Verification items for the finished model (mm, model axes). A direction names the side the tool comes from. Round coordinates to 2 decimals unless told otherwise and drop trailing zeros. Order: outer loops, then holes, each group sorted by start corner. A loop starts at its lowest first (then second) coordinate and runs counter-clockwise, first axis right, second up.
```python
from build123d import *

# Parameters (mm, degrees)
F0_R      = 3.5
F1_DEPTH  = 1.5
F2_R      = 2.5
F3_DEPTH  = 1
F4_R      = 3.5
F4_R_2    = 2.5
F5_DEPTH  = 1.5
F6_R      = 1
F7_R      = 1
F10_R     = 3.5
F11_DEPTH = 1.5
F12_R     = 1
F13_D     = 3.5


with BuildPart() as f1:
    # F0 (on Front) → F1 (new body)
    with BuildSketch(Plane.XZ):
        Circle(F0_R)
    extrude(amount=F1_DEPTH)

    # F2 (on face) → F3 (join)
    with BuildSketch(Plane.XZ.offset(1.5)):
        Circle(F2_R)
    extrude(amount=F3_DEPTH)

    # F7
    f7_edges = [f1.edges().sort_by_distance(p)[0] for p in [
        (-3.5, 0, 0),
    ]]
    fillet(f7_edges, radius=F7_R)

    # F10 (on face) → F11 (join)
    with BuildSketch(Plane.XZ.offset(2.5)):
        Circle(F10_R)
    extrude(amount=F11_DEPTH)

    # F12
    f12_edges = [f1.edges().sort_by_distance(p)[0] for p in [
        (-3.5, -4, 0),
    ]]
    fillet(f12_edges, radius=F12_R)

    # F13 (through all)
    with Locations(Plane.XZ.offset(4)):
        with Locations((0, 0)):
            Hole(F13_D / 2)


with BuildPart() as f5:
    # F4 (on face) → F5 (new body)
    with BuildSketch(Plane.XZ.offset(2.5)):
        Circle(F4_R)
        Circle(F4_R_2, mode=Mode.SUBTRACT)
        Circle(F4_R_2)
    extrude(amount=F5_DEPTH)

    # F6
    f6_edges = [f5.edges().sort_by_distance(p)[0] for p in [
        (-3.5, -4, 0),
    ]]
    fillet(f6_edges, radius=F6_R)


solid = f1.part
```
1) Draft check along X on faces 3 (the cylindrical face through (-1.617, -1.972, -0.67)), 4 (the flat face through (2, -1.5, -2)), 5 (the cylindrical face through (3.233, -1.246, -1.341)). Enter one of: released by +X, released by -X, zero draft, split by the parting line, or undercut.
2) Tool access check on faces 1 (the flat face through (1, -4, 2)), 2 (the flat face through (2, -2.5, -2)). Record the directions out of +Z, -Z, +X, -X, +Y, -Y that give a thin tool (end or side, any length) a straight path to the whole face; none if there is none.
3) Sectioned sample at C-C on y = -1.65. Record the cut outline in (x, z).
4) Sectioned sample at A-A on z = 0. Record the cut outline in (x, y).
5) Sectioned sample at B-B on x = 0. Record the cut outline in (y, z).
6) Scan lines: probe 1 along Z at (x, y) = (0, -0.95); probe 2 along Z at (x, y) = (0, -1.9); probe 3 along Y at (x, z) = (2.75, -0.75). Record each from-to range of solid material in increasing order.
7) Go/stop test with flat-tipped pins: pin 1 Ø1.5 at (x, y) = (2.5, -0.5) entering from +Z; pin 2 Ø3 at (x, z) = (0, 0) entering from -Y; pin 3 Ø3 at (x, z) = (-1, 2.5) entering from -Y; pin 4 Ø1 at (y, z) = (-3, 2) entering from +X. Record where each tip stops, or that it passes through.
Returned:
1. face 3: undercut
1. face 4: zero draft
1. face 5: split by the parting line
2. face 1: +Z, -Z, +X, -X, -Y
2. face 2: none
3. outline: circle Ø5 at (0, 0); hole circle Ø3.5 at (0, 0)
4. outline: (-3.5, -3) arc R1 ccw to (-2.5, -4) - (-1.75, -4) - (-1.75, 0) - (-2.5, 0) arc R1 ccw to (-3.5, -1) - (-3.5, -1.5) - (-2.5, -1.5) - (-2.5, -2.5) - (-3.5, -2.5) - close; (1.75, -4) - (2.5, -4) arc R1 ccw to (3.5, -3) - (3.5, -2.5) - (2.5, -2.5) - (2.5, -1.5) - (3.5, -1.5) - (3.5, -1) arc R1 ccw to (2.5, 0) - (1.75, 0) - close
5. outline: (-4, -2.5) arc R1 ccw to (-3, -3.5) - (-2.5, -3.5) - (-2.5, -2.5) - (-1.5, -2.5) - (-1.5, -3.5) - (-1, -3.5) arc R1 ccw to (0, -2.5) - (0, -1.75) - (-4, -1.75) - close; (-4, 1.75) - (0, 1.75) - (0, 2.5) arc R1 ccw to (-1, 3.5) - (-1.5, 3.5) - (-1.5, 2.5) - (-2.5, 2.5) - (-2.5, 3.5) - (-3, 3.5) arc R1 ccw to (-4, 2.5) - close
6. probe 1: z = -3.5 to -1.75, 1.75 to 3.5
6. probe 2: z = -2.5 to -1.75, 1.75 to 2.5
6. probe 3: y = -3.94 to -2.5, -1.5 to -0.06
7. pin 1: stops at z = 2.97
7. pin 2: passes through
7. pin 3: stops at y = -4
7. pin 4: stops at x = 3.16
